Work out the finished part from the listing and answer in its coordinate system (mm). Face numbers are marked on the shaded views. A direction names the side the tool comes from. Give positions to 0.01 mm unless a question says otherwise; leave off trailing zeros. Loops run counter-clockwise (first coordinate to the right, second up) from the corner with the lowest first, then second, coordinate; pieces in that order, holes last. Notation, with made-up numbers: (72, 32.25) - (112, 32.25) arc R34 ccw to (112, 67.25) - close; hole circle Ø9 at (1.5, 89). An arc over 180 degrees is marked (long way). Use CSV: the item, a comma, the result in double quotes.
from build123d import *

# Parameters (mm, degrees)
TONGUE_SKETCH_W   = 27
TONGUE_SKETCH_H   = 22
TONGUE_DEPTH      = 7
PAD_SKETCH_W      = 6
PAD_SKETCH_H      = 8
SWITCH_PAD_DEPTH  = 19
PIN_HOLE_SKETCH_R = 3.1
PIN_HOLE_DEPTH    = 10


with BuildPart() as part:
    # Stem Sketch → Stem (revolve)
    with BuildSketch(Plane.XY, mode=Mode.PRIVATE) as stem_sk:
        Polygon((14, 0), (14, 15), (20, 15), (20, 13.45), (65, 13.45), (65, 11), (30, 11), (30, 0), align=None)
    revolve(stem_sk.sketch.rotate(Axis((-3000, 0, 0), (1, 0, 0)), 90), axis=Axis((-3000, 0, 0), (1, 0, 0)))

    # Tongue Sketch → Tongue (add, symmetric)
    with BuildSketch(Plane.XY):
        with Locations((2.5, 0)):
            Rectangle(TONGUE_SKETCH_W, TONGUE_SKETCH_H)
    extrude(amount=TONGUE_DEPTH, both=True)

    # Pad Sketch → Switch Pad (add, symmetric)
    with BuildSketch(Plane.XY):
        with Locations((17, 13)):
            Rectangle(PAD_SKETCH_W, PAD_SKETCH_H)
    extrude(amount=SWITCH_PAD_DEPTH, both=True)

    # Pin Hole Sketch → Pin Hole (cut, symmetric)
    with BuildSketch(Plane.XY):
        Circle(PIN_HOLE_SKETCH_R)
    extrude(amount=PIN_HOLE_DEPTH, both=True, mode=Mode.SUBTRACT)


solid = part.part
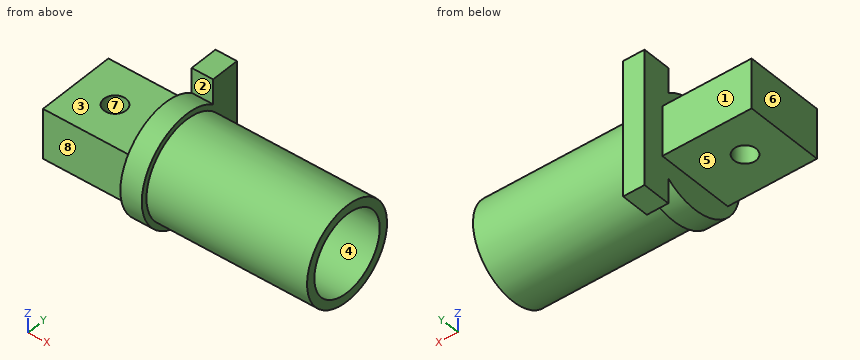
Item 1: A cutting plane is placed at A-A on x = 0. Determine the outline of the cut face in (y, z).
Determined:
outline,"(-11, -7) - (-3.1, -7) - (-3.1, 7) - (-11, 7) - close; (3.1, -7) - (11, -7) - (11, 7) - (3.1, 7) - close"
Item 2: For the marked faces 1, 2, 3, 4 and 5, determine the directions among +Z, -Z, +X, -X, +Y, -Y from which every point of the face is accessible in a straight line to the end or side of a thin tool.
Determined:
face 1,"+Z, -Z, -X, +Y"
face 2,"+Z, +X, -X"
face 3,"+Z, -X, +Y, -Y"
face 4,"+X"
face 5,"-Z, -X, +Y, -Y"
Item 3: A cutting plane is placed at D-D on x = 55. Determine the outline of the cut face in (y, z).
Determined:
outline,"circle Ø26.9 at (0, 0); hole circle Ø22 at (0, 0)"
Item 4: A cutting plane is placed at B-B on y = 0. Determine the outline of the cut face in (x, z), and give its area (3 significant figures).
Determined:
outline,"(-11, -7) - (-3.1, -7) - (-3.1, 7) - (-11, 7) - close; (3.1, -7) - (14, -7) - (14, -15) - (20, -15) - (20, -13.45) - (65, -13.45) - (65, -11) - (30, -11) - (30, 11) - (65, 11) - (65, 13.45) - (20, 13.45) - (20, 15) - (14, 15) - (14, 7) - (3.1, 7) - close"
area,"884 mm²"
Item 5: Find the intervals of material crossed by line 1 (Y direction, x = 46, z = 0); line 2 (Y direction, x = 0, z = -0.75); line 3 (Y direction, x = -3.5, z = 3), in increasing order.
Determined:
line 1,"y = -13.45 to -11, 11 to 13.45"
line 2,"y = -11 to -3.1, 3.1 to 11"
line 3,"y = -11 to 11"
Item 6: Given P1, Ø4, axis at x = 15, z = -8.5, coming from the -Y side; P2, Ø3, axis at x = 47, y = 10, coming from the -Z side; P3, Ø8, axis at x = 57, y = -0.5, coming from the +Z side, each flat-ended and moving along its own axis, determine where each tip first touches the part or whether it passes through.
Determined:
P1,"stops at y = -13.52"
P2,"stops at z = -10.42"
P3,"stops at z = 13.45"
Item 7: A cutting plane is placed at C-C on z = 0. Determine the outline of the cut face in (x, y).
Determined:
outline,"(-11, -11) - (14, -11) - (14, -15) - (20, -15) - (20, -13.45) - (65, -13.45) - (65, -11) - (30, -11) - (30, 11) - (65, 11) - (65, 13.45) - (20, 13.45) - (20, 17) - (14, 17) - (14, 11) - (-11, 11) - close; hole circle Ø6.2 at (0, 0)"
Item 8: The mould has two halves that part along X. Classify the marked faces 6, 7 and 8: pulls with the +X half, pulls with the -X half, needs draft (parallel to the pull), parting line crosses it, or undercut.
Determined:
face 6,"pulls with the -X half"
face 7,"undercut"
face 8,"needs draft"
